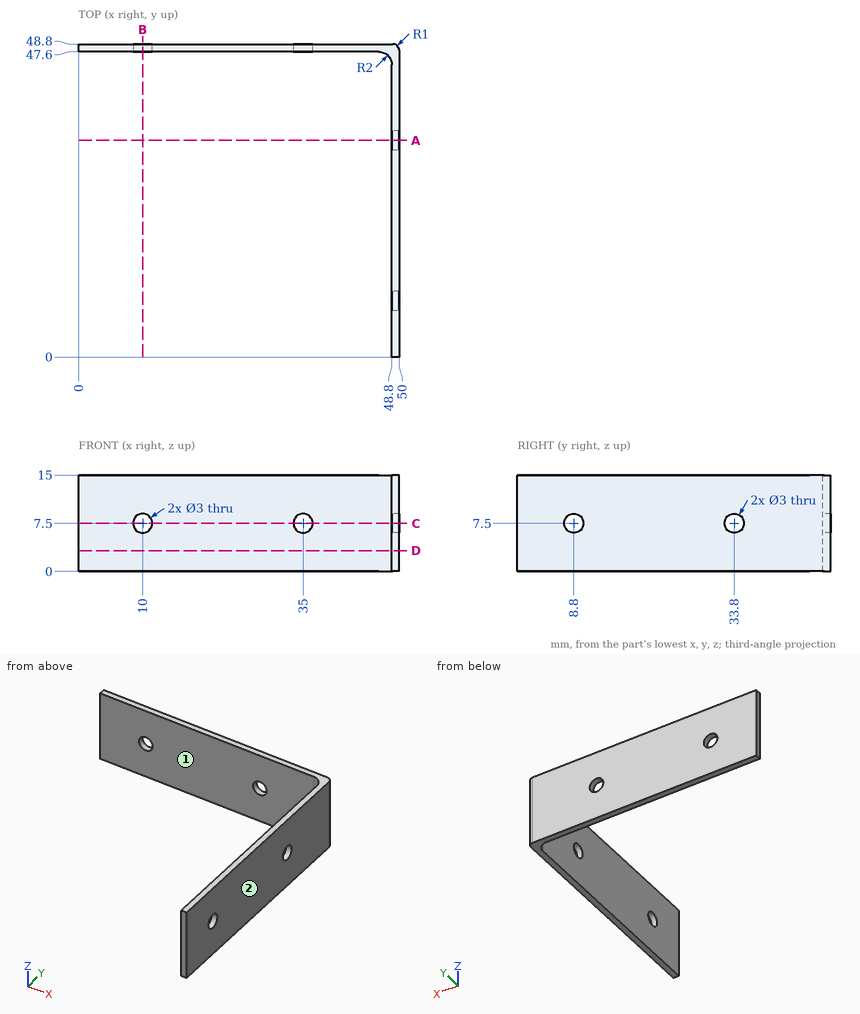
Print and shaded views of the part. All mm, measured from the part's lowest x, y and z. A direction names the side the tool comes from. Give positions to 0.01 mm unless a question says otherwise; leave off trailing zeros. Loops run counter-clockwise (first coordinate to the right, second up) from the corner with the lowest first, then second, coordinate; pieces in that order, holes last. Notation, with made-up numbers: M 7,-10.75 L 51,-10.75 A12 ccw 51,-2.75 Z; hole C 24.25,69.5 d2. An arc over 180 degrees is marked long. Write each question's results on one line, items separated by ' | '.
Q1. Flat gauge pins, fed straight in: P1, Ø4, axis at y = 8.8, z = 7.5, coming from the -X side; P2, Ø7.5, axis at x = 27, z = 4, coming from the -Y side. Where does each tip first touch, or does it go through?
Geometry check:
P1: stops at x = 48.8 | P2: stops at y = 47.6
Q2. Band-saw the part on B-B on x = 10. Write the cut outline in (y, z), and give its area (3 significant figures).
Geometry check:
outline: M 47.6,0 L 48.8,0 L 48.8,6 L 47.6,6 Z; M 47.6,9 L 48.8,9 L 48.8,15 L 47.6,15 Z | area: 14.4 mm²
Q3. Band-saw the part on A-A on y = 33.8. Write the cut outline in (x, z).
Geometry check:
outline: M 48.8,0 L 50,0 L 50,6 L 48.8,6 Z; M 48.8,9 L 50,9 L 50,15 L 48.8,15 Z
Q4. Probe probe 1 along Z at (x, y) = (35, 48); probe 2 along X at (y, z) = (22.5, 8); probe 3 along Y at (x, z) = (22.5, 8.5). List the from-to ranges inside material, lowest first.
Geometry check:
probe 1: z = 0 to 6, 9 to 15 | probe 2: x = 48.8 to 50 | probe 3: y = 47.6 to 48.8
Q5. Band-saw the part on D-D on z = 3.25. Write the cut outline in (x, y).
Geometry check:
outline: M 0,47.6 L 46.8,47.6 A2 cw 48.8,45.6 L 48.8,0 L 50,0 L 50,47.8 A1 ccw 49,48.8 L 0,48.8 Z
Q6. Which spindle directions (+Z, -Z, +X, -X, +Y, -Y) get a long thin tool onto all of the face, cutting with end or side? Do the marked faces 1 and 2. Say none if no direction does.
Geometry check:
face 1: +Z, -Z, -X, -Y | face 2: +Z, -Z, +X, +Y, -Y
Q7. Band-saw the part on C-C on z = 7.5. Write the cut outline in (x, y), and give its area (3 significant figures).
Geometry check:
outline: M 0,47.6 L 8.5,47.6 L 8.5,48.8 L 0,48.8 Z; M 11.5,47.6 L 33.5,47.6 L 33.5,48.8 L 11.5,48.8 Z; M 36.5,47.6 L 46.8,47.6 A2 cw 48.8,45.6 L 48.8,35.3 L 50,35.3 L 50,47.8 A1 ccw 49,48.8 L 36.5,48.8 Z; M 48.8,0 L 50,0 L 50,7.3 L 48.8,7.3 Z; M 48.8,10.3 L 50,10.3 L 50,32.3 L 48.8,32.3 Z | area: 103 mm²
